Read the model definition and answer for the solid it produces. Units are mm, in the model's axes. Round coordinates to 2 decimals unless told otherwise and drop trailing zeros. Order: outer loops, then holes, each group sorted by start corner. A loop starts at its lowest first (then second) coordinate and runs counter-clockwise, first axis right, second up.
from build123d import *

# Parameters (mm, degrees)
F0_W     = 50
F0_H     = 50
F1_DEPTH = 50
F1_TAPER = 30


with BuildPart() as f1:
    # F0 (on Top) → F1 (new body)
    with BuildSketch(Plane.XY):
        Rectangle(F0_W, F0_H)
    extrude(amount=F1_DEPTH, taper=F1_TAPER)

    # F2: F1 across plane


with BuildPart() as f1_1:
    add(f1.part)
    add(f1.part.mirror(Plane.XY))


solid = f1_1.part
Q1. Flat-ended cylindrical pins translate along their axes: pin 1 (2 mm diameter, centred on x = -17, y = 10.5, fed in from +Z); pin 2 (12 mm diameter, centred on y = 16, z = 29, fed in from +X); pin 3 (5 mm diameter, centred on x = -16, y = -2, fed in from +Z); pin 4 (5 mm diameter, centred on x = -12.5, y = 15, fed in from +Z). Find the tip coordinate at first contact, or state that the pin passes through.
Outcome:
pin 1: stops at z = 15.59
pin 2: passes through
pin 3: stops at z = 19.92
pin 4: stops at z = 21.65
Q2. Straight lines are drawn through the part: probe 1 along Z at (x, y) = (2, -17); probe 2 along Y at (x, z) = (13, 13.5). For each, find the intervals that lie inside material, in ascending order.
Outcome:
probe 1: z = -13.86 to 13.86
probe 2: y = -17.21 to 17.21
Q3. A cutting plane is placed at D-D, the plane z = -10. Give the vertices of the cut face in (x, y), plus the area to 3 significant figures.
Outcome:
outline: (-19.23, -19.23) - (19.23, -19.23) - (19.23, 19.23) - (-19.23, 19.23) - close
area: 1,480 mm2
Q4. A cutting plane is placed at A-A, the plane y = -9. Give the vertices of the cut face in (x, z).
Outcome:
outline: (-25, 0) - (-9, -27.71) - (9, -27.71) - (25, 0) - (9, 27.71) - (-9, 27.71) - close
Q5. A cutting plane is placed at B-B, the plane x = 15. Give the vertices of the cut face in (y, z).
Outcome:
outline: (-25, 0) - (-15, -17.32) - (15, -17.32) - (25, 0) - (15, 17.32) - (-15, 17.32) - close
Q6. A cutting plane is placed at C-C, the plane z = -31. Give the vertices of the cut face in (x, y), plus the area to 3 significant figures.
Outcome:
outline: (-7.1, -7.1) - (7.1, -7.1) - (7.1, 7.1) - (-7.1, 7.1) - close
area: 202 mm2
